from build123d import *

# Parameters (mm, degrees)
SKETCH2_W           = 6
SKETCH2_H           = 4
BOSS_EXTRUDE1_DEPTH = 5
SKETCH3_W           = 1
SKETCH3_H           = 3
CUT_EXTRUDE1_DEPTH  = 5
CUT_EXTRUDE2_DEPTH  = 3


with BuildPart() as part:
    # Sketch2 → Boss-Extrude1 (new body)
    with BuildSketch(Plane(origin=(0, 0, 0), x_dir=(1, 0, 0), z_dir=(0, 1, 0))):
        with Locations((3, 2)):
            Rectangle(SKETCH2_W, SKETCH2_H)
    extrude(amount=BOSS_EXTRUDE1_DEPTH)

    # Sketch3 → Cut-Extrude1 (cut)
    with BuildSketch(Plane.XY):
        Polygon((0, 5), (0, 3), (2, 5), align=None)
        with Locations((0.5, 1.5)):
            Rectangle(SKETCH3_W, SKETCH3_H)
    extrude(amount=-CUT_EXTRUDE1_DEPTH, mode=Mode.SUBTRACT)

    # Sketch4 → Cut-Extrude2 (cut)
    with BuildSketch(Plane.XZ):
        Polygon((1, -4), (4, 0), (1, 0), align=None)
    extrude(amount=-CUT_EXTRUDE2_DEPTH, mode=Mode.SUBTRACT)


solid = part.part
Model file for the job. Use its own axes, mm. A direction names the side the tool comes from. Round coordinates to 2 decimals unless told otherwise and drop trailing zeros. Loops run counter-clockwise (first coordinate to the right, second up) from the corner with the lowest first, then second, coordinate; pieces in that order, holes last. Notation, with made-up numbers: (-40, 2.25) -> (-11, 2.25) arc R25 ccw to (-11, 32.25) -> close; hole circle Ø7 at (65.25, -34.5). An arc over 180 degrees is marked (long way). Answer as CSV lines item,"result". Start each with the question number.
1) Slice it at A-A (x = 1.3). List the corners of the cut face in (y, z), plus the area to 3 significant figures.
2) Slice it at B-B (z = -0.4). List the corners of the cut face in (x, y).
3) Slice it at D-D (y = 3.15). List the corners of the cut face in (x, z).
4) Probe line 1 along X through (y, z) = (4, -2.85); line 2 along Y through (x, z) = (2.65, -1.15); line 3 along Z through (x, y) = (1.2, 0.65). List the from-to ranges inside material, lowest first.
5) Pin check, flat tip, straight feed: P1, Ø2, axis at x = 3, y = 2.5, coming from the +Z side. Stop position of the tip, or through.
6) Slice it at C-C (y = 1.2). List the corners of the cut face in (x, z), plus the area to 3 significant figures.
7) Tool access for faces 1 (the face through (1, 4, -2)), 2 (the face through (2, 3, -2)): list every direction of +Z, -Z, +X, -X, +Y, -Y with a clear straight run to the whole face (end or side of a thin tool).
Filled in:
1,outline,"(0, -4) -> (4.3, -4) -> (4.3, 0) -> (3, 0) -> (3, -3.6) -> (0, -3.6) -> close"
1,area,"6.40 mm2"
2,outline,"(0, 3) -> (3.7, 3) -> (3.7, 0) -> (6, 0) -> (6, 5) -> (2, 5) -> close"
3,outline,"(0.15, -4) -> (6, -4) -> (6, 0) -> (0.15, 0) -> close"
4,line 1,"x = 1 to 6"
4,line 2,"y = 3 to 5"
4,line 3,"z = -4 to -3.73"
5,P1,"stops at z = 0"
6,outline,"(1, -4) -> (6, -4) -> (6, 0) -> (4, 0) -> close"
6,area,"14.0 mm2"
7,face 1,"+Z, -Z, -X, +Y"
7,face 2,"+Z, -X, -Y"
